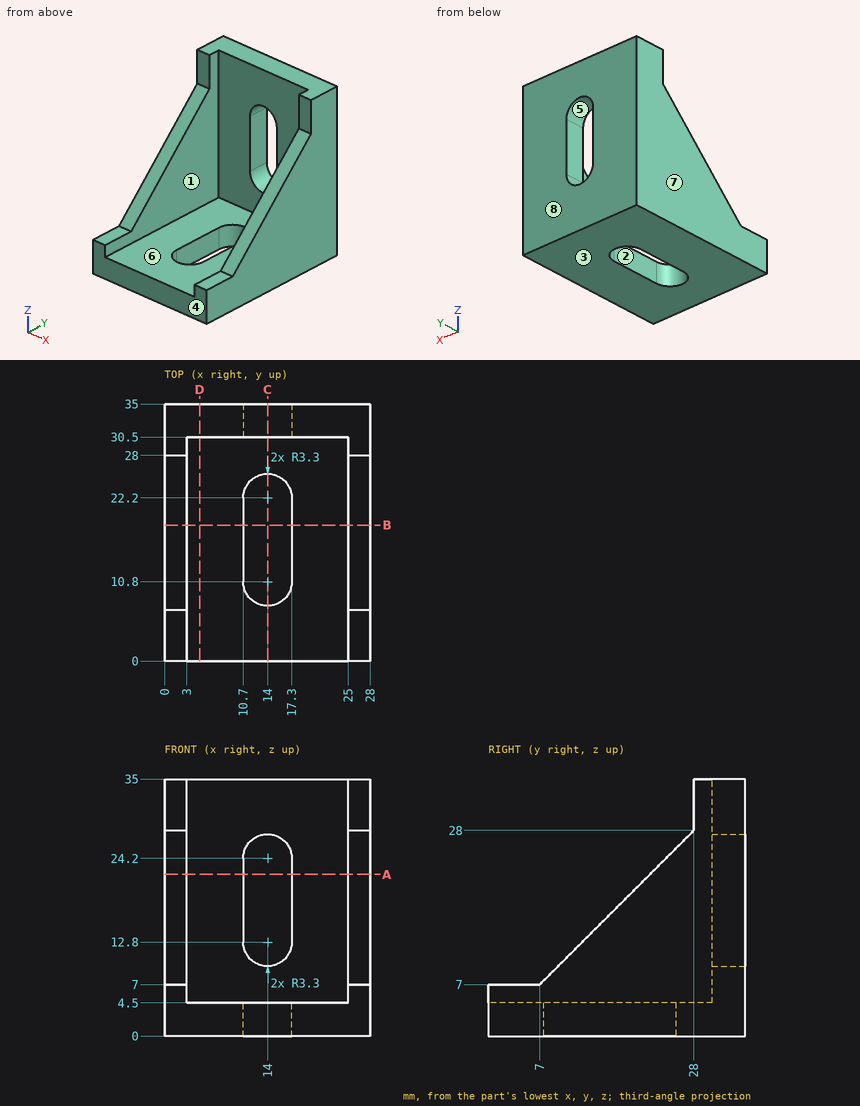
Part print with two shaded views. Sizes in mm from the minimum x, y, z corner. A direction names the side the tool comes from. Round coordinates to 2 decimals unless told otherwise and drop trailing zeros. Order: outer loops, then holes, each group sorted by start corner. A loop starts at its lowest first (then second) coordinate and runs counter-clockwise, first axis right, second up. Notation, with made-up numbers: (74, -33) - (109, -33) arc R30 ccw to (109, -8) - close; hole circle Ø9 at (46, -18.5). An arc over 180 degrees is marked (long way). Return JSON: item names as keys, results as strings.
(1) Pull direction X, two halves, no side cores. Call the marked faces 6, 7 and 8: +X half, -X half, draft (parallel to the pull), parting line (faces both ways), or undercut.
Answer key:
{"face 6": "undercut", "face 7": "-X half", "face 8": "draft"}
(2) Tool access for the marked faces 1, 2, 3, 4 and 5: list every direction of +Z, -Z, +X, -X, +Y, -Y with a clear straight run to the whole face (end or side of a thin tool).
Answer key:
{"face 1": "+Z, -Y", "face 2": "+Z, -Z", "face 3": "-Z, +X, -X, +Y, -Y", "face 4": "+Z, -Z, +X, -X, -Y", "face 5": "+Y, -Y"}
(3) Wall check: probe 1 along X at (y, z) = (30, 9); probe 2 along Z at (x, y) = (12.25, 7.5); probe 3 along Y at (x, z) = (9.5, 29). Give the ranges that are in metal, low to high. Write a range as from..to.
Answer key:
{"probe 1": "x = 0..3, 25..28", "probe 2": "z = 0..4.5", "probe 3": "y = 30.5..35"}
(4) Cut at A-A (z = 22). Give the cut face in (x, y), then the cut area to 3 significant figures.
Answer key:
{"outline": "(0, 22) - (3, 22) - (3, 30.5) - (10.7, 30.5) - (10.7, 35) - (0, 35) - close; (17.3, 30.5) - (25, 30.5) - (25, 22) - (28, 22) - (28, 35) - (17.3, 35) - close", "area": "147 mm^2"}
(5) Cut at D-D (x = 4.75). Give the cut face in (y, z).
Answer key:
{"outline": "(0, 0) - (35, 0) - (35, 35) - (30.5, 35) - (30.5, 4.5) - (0, 4.5) - close"}
(6) Cut at B-B (y = 18.5). Give the cut face in (x, z).
Answer key:
{"outline": "(0, 0) - (10.7, 0) - (10.7, 4.5) - (3, 4.5) - (3, 18.5) - (0, 18.5) - close; (17.3, 0) - (28, 0) - (28, 18.5) - (25, 18.5) - (25, 4.5) - (17.3, 4.5) - close"}
(7) Pin check, flat tips, straight feed: pin 1 Ø3.5 at (x, y) = (27, 4.5) entering from +Z; pin 2 Ø6.5 at (x, z) = (11, 17.5) entering from -Y; pin 3 Ø0.9 at (x, z) = (1, 33) entering from -Y. Stop position of each tip, or through.
Answer key:
{"pin 1": "stops at z = 7", "pin 2": "stops at y = 30.5", "pin 3": "stops at y = 28"}
(8) Cut at C-C (x = 14). Give the cut face in (y, z).
Answer key:
{"outline": "(0, 0) - (7.5, 0) - (7.5, 4.5) - (0, 4.5) - close; (25.5, 0) - (35, 0) - (35, 9.5) - (30.5, 9.5) - (30.5, 4.5) - (25.5, 4.5) - close; (30.5, 27.5) - (35, 27.5) - (35, 35) - (30.5, 35) - close"}
